from build123d import *

# Parameters (mm, degrees)
SKETCH1_R           = 10
BOSS_EXTRUDE1_DEPTH = 25
SKETCH2_W           = 0.8
SKETCH2_H           = 5
BOSS_EXTRUDE2_DEPTH = 8
BOSS_EXTRUDE3_DEPTH = 1.2
CUT_EXTRUDE1_DEPTH  = 25
SKETCH6_W           = 5
SKETCH6_H           = 8
BOSS_EXTRUDE4_DEPTH = 0.8
CUT_EXTRUDE2_REACH  = 29.411


with BuildPart() as part:
    # Sketch1 → Boss-Extrude1 (new body)
    with BuildSketch(Plane(origin=(0, 0, 0), x_dir=(1, 0, 0), z_dir=(0, 1, 0))):
        with Locations(Location((0, 0, 0), (0, 0, 270))):
            Circle(SKETCH1_R)
    extrude(amount=BOSS_EXTRUDE1_DEPTH)

    # Sketch5 → Cut-Extrude1 (cut)
    with BuildSketch(Plane.XZ):
        with BuildLine():
            Line((-8.64, -5.034918073), (8.64, -5.034918073))
            ThreePointArc((8.64, -5.034918073), (0, -10), (-8.64, -5.034918073))
        make_face()
        with BuildLine():
            Line((-8.64, 5.034918073), (8.64, 5.034918073))
            ThreePointArc((8.64, 5.034918073), (0, 10), (-8.64, 5.034918073))
        make_face()
    extrude(amount=-CUT_EXTRUDE1_DEPTH, mode=Mode.SUBTRACT)



with BuildPart() as body_2:
    # Sketch2 → Boss-Extrude2 (new body)
    with BuildSketch(Plane(origin=(0, 0, 0), x_dir=(-1, 0, 0), z_dir=(0, -1, 0))):
        with Locations((7.65, 0)):
            Rectangle(SKETCH2_W, SKETCH2_H)
    extrude(amount=BOSS_EXTRUDE2_DEPTH)

    # Sketch3 → Boss-Extrude3 (add)
    with BuildSketch(Plane.ZY.offset(8.05)):
        Polygon((-2.5, -8), (-2.5, 0), (2.5, 0), (2.5, -8), (1.5, -8), (1.5, -0.75), (-1.5, -0.75), (-1.5, -8), align=None)
    extrude(amount=BOSS_EXTRUDE3_DEPTH)


with BuildPart() as part_1:
    add(part.part)

    add(body_2.part)  # Boss-Extrude4 merges body 2
    # Sketch6 → Boss-Extrude4 (add)
    with BuildSketch(Plane.ZY.offset(9.25)):
        with Locations((0, -4)):
            Rectangle(SKETCH6_W, SKETCH6_H)
    extrude(amount=BOSS_EXTRUDE4_DEPTH)

    # Sketch7 → Cut-Extrude2 (cut, up to next)
    with BuildSketch(Plane(origin=(0, 0, 0), x_dir=(1, 0, 0), z_dir=(0, 1, 0)), mode=Mode.PRIVATE) as cut_extrude2_sk1:
        with BuildLine():
            Line((-9.682458366, 2.5), (-10.05, 2.5))
            Line((-10.05, 2.5), (-10.05, -2.5))
            Line((-10.05, -2.5), (-9.682458366, -2.5))
            ThreePointArc((-9.682458366, -2.5), (-10, 0), (-9.682458366, 2.5))
        make_face()
    cut_extrude2_tool1 = extrude(cut_extrude2_sk1.sketch, amount=-CUT_EXTRUDE2_REACH, mode=Mode.PRIVATE) & part_1.part
    add(cut_extrude2_tool1.solids().sort_by_distance((-9.866229, 0, -2.449865))[0], mode=Mode.SUBTRACT)


solid = part_1.part
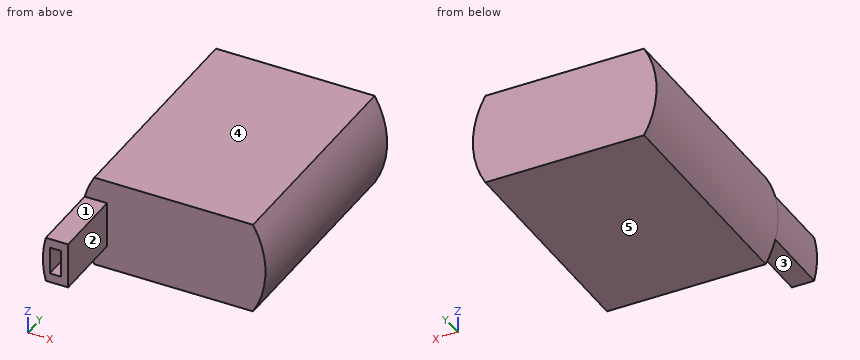
Can you work these out from the model? Positions are in its coordinate system, mm. Face numbers are marked on the shaded views. A direction names the side the tool comes from. Coordinates: 2 decimals unless noted, no trailing zeros. Order: outer loops, then holes, each group sorted by start corner. A loop starts at its lowest first (then second) coordinate and runs counter-clockwise, first axis right, second up. Notation, with made-up numbers: M -8.5,-4.75 L 28.5,-4.75 A17 cw 28.5,10.25 Z; hole C 78,10 d4. An arc over 180 degrees is marked long. Write item = value, one per line.
(1) Suppose I cut it at B-B on z = 2. Please give me the cut outline in (x, y), plus the area to 3 significant figures.
Results are:
outline = M -9.8,-8 L -7.25,-8 L -7.25,0 L 9.8,0 L 9.8,25 L -9.8,25 Z
area = 510 mm2
(2) I need wall thicknesses on line 1 along Y through (x, z) = (2, -2); line 2 along X through (y, z) = (-2.5, 1.25); line 3 along X through (y, z) = (6, 2.5). Which ranges of each line are inside material? Lowest first, please. Write a range as [from, to].
Results are:
line_1 = [0, 25]
line_2 = [-9.92, -9.25], [-8.05, -7.25]
line_3 = [-9.68, 9.68]
(3) For the marked faces 1, 2, 3, 4 and 5, which set-ups out of +Z, -Z, +X, -X, +Y, -Y let a thin tool reach every point of the face, with its end or its side?
Results are:
face_1 = +Z, +X, -X, -Y
face_2 = +Z, -Z, +X, -Y
face_3 = -Z, +X, -X, -Y
face_4 = +Z, +X, -X, +Y, -Y
face_5 = -Z, +X, -X, +Y, -Y
(4) Suppose I cut it at C-C on x = 7. Please give me the cut outline in (y, z), plus the area to 3 significant figures.
Results are:
outline = M 0,-5.03 L 25,-5.03 L 25,5.03 L 0,5.03 Z
area = 252 mm2
(5) Suppose I cut it at D-D on y = 14.5. Please give me the cut outline in (x, z).
Results are:
outline = M -8.64,-5.03 L 8.64,-5.03 A10 ccw 8.64,5.03 L -8.64,5.03 A10 ccw Z
(6) Suppose I cut it at A-A on y = -4. Please give me the cut outline in (x, z), plus the area to 3 significant figures.
Results are:
outline = M -9.68,-2.5 L -7.25,-2.5 L -7.25,2.5 L -9.68,2.5 A10 ccw Z; hole M -9.25,-1.5 L -8.05,-1.5 L -8.05,1.5 L -9.25,1.5 Z
area = 9.62 mm2
(7) For pin 1 Ø0.7 at (x, y) = (-8.5, -3) entering from -Z; pin 2 Ø2.5 at (y, z) = (-3, 0.5) entering from +X; pin 3 Ø1.9 at (x, y) = (-9, -3.5) entering from +Z, each with a flat end and sliding along its axis, tell me the tip position at first contact or that it passes through.
Results are:
pin_1 = -2.5
pin_2 = -7.25
pin_3 = 2.5
